from build123d import *

# Parameters (mm, degrees)
SKETCH1_R           = 11
BOSS_EXTRUDE1_DEPTH = 4
SKETCH5_R           = 5
SKETCH5_R_2         = 2
BOSS_EXTRUDE2_DEPTH = 15
SKETCH2_R           = 1.25
CUT_EXTRUDE1_DEPTH  = 10
SKETCH20_R          = 1.25
CUT_EXTRUDE2_DEPTH  = 4


with BuildPart() as part:
    # Sketch1 → Boss-Extrude1 (new body)
    with BuildSketch(Plane(origin=(0, 0, 0), x_dir=(1, 0, 0), z_dir=(0, 1, 0))):
        with Locations(Location((0, 0, 0), (0, 0, 270))):
            Circle(SKETCH1_R)
    extrude(amount=BOSS_EXTRUDE1_DEPTH)

    # Sketch5 → Boss-Extrude2 (add)
    with BuildSketch(Plane.XZ):
        with Locations(Location((0, 0, 0), (0, 0, 90))):
            Circle(SKETCH5_R)
        with Locations(Location((0, 0, 0), (0, 0, 270))):
            Circle(SKETCH5_R_2, mode=Mode.SUBTRACT)
    extrude(amount=BOSS_EXTRUDE2_DEPTH)

    # Sketch2 → Cut-Extrude1 (cut)
    with BuildSketch(Plane.XZ):
        with Locations(Location((0, -8, 0), (0, 0, 270))):
            Circle(SKETCH2_R)
        with Locations(Location((-8, 0, 0), (0, 0, 270))):
            Circle(SKETCH2_R)
        with Locations(Location((0, 8, 0), (0, 0, 270))):
            Circle(SKETCH2_R)
        with Locations(Location((8, 0, 0), (0, 0, 270))):
            Circle(SKETCH2_R)
    extrude(amount=-CUT_EXTRUDE1_DEPTH, mode=Mode.SUBTRACT)

    # Sketch20 → Cut-Extrude2 (cut)
    with BuildSketch(Plane(origin=(5, 0, 0), x_dir=(0, 0, -1), z_dir=(1, 0, 0))):
        with Locations((0, -4)):
            Circle(SKETCH20_R)
        with Locations((0, -11)):
            Circle(SKETCH20_R)
    extrude(amount=-CUT_EXTRUDE2_DEPTH, mode=Mode.SUBTRACT)


solid = part.part
The model under review builds one solid part; all positions refer to its coordinate system, in mm. A direction names the side the tool comes from. Give positions to 0.01 mm unless a question says otherwise; leave off trailing zeros. Loops run counter-clockwise (first coordinate to the right, second up) from the corner with the lowest first, then second, coordinate; pieces in that order, holes last. Notation, with made-up numbers: (55, 80) -> (72, 80) arc R20 ccw to (72, 107) -> close; hole circle Ø5 at (59.5, 32.5). An arc over 180 degrees is marked (long way). Answer as a JSON object with one key per item and string values. Group by question number.
Q1. Take a section at C-C (z = 8). Write out the cut boundary in (x, y).
Q2. Tool access review of faces 1 (the cylindrical face through (3.3, -10.95, 1.25)), 2 (the flat face through (0, 0, 0)), 3 (the flat face through (0, 4, 0)): name each direction out of +Z, -Z, +X, -X, +Y, -Y from which nothing blocks a thin tool from reaching the whole face with its end or side.
Q3. Take a section at A-A (x = 0). Write out the cut boundary in (y, z).
Q4. Draft analysis for pull direction Y (two halves, no side actions). For faces 4 (the cylindrical face through (0.05, 1.97, 9.25)), 5 (the cylindrical face through (3.3, -3.95, 1.25)), 6 (the flat face through (-0.1, -15, 2.2)), state which applies: pulls with the +Y half, pulls with the -Y half, needs draft (parallel to the pull), parting line crosses it, or undercut.
Q5. Take a section at B-B (x = 8). Write out the cut boundary in (y, z).
Q6. Insertion check: pin 1 (1.5 mm diameter, centred on y = -2.5, z = -1, fed in from -X); pin 2 (1.5 mm diameter, centred on x = 7, y = 1.5, fed in from +Z); pin 3 (3 mm diameter, centred on x = -8, z = 0, fed in from -Y); pin 4 (2 mm diameter, centred on x = 8, z = 0, fed in from +Y). Each pin has a flat end and moves straight along its axis. Give the tip position at first contact, or say it passes through.
Q7. Wall thickness on line 1 along X through (y, z) = (1.35, 0); line 2 along Y through (x, z) = (-6.5, 6.25); line 3 along X through (y, z) = (2.35, 8): over which ranges is each line inside the solid? List them lowest first.
Q8. Take a section at D-D (y = -7). Write out the cut boundary in (x, z).
Answer below:
{
 "1": {"outline": "(-7.55, 0) -> (-1.25, 0) -> (-1.25, 4) -> (-7.55, 4) -> close; (1.25, 0) -> (7.55, 0) -> (7.55, 4) -> (1.25, 4) -> close"},
 "2": {"face 1": "+X", "face 2": "-Y", "face 3": "+Z, -Z, +X, -X, +Y"},
 "3": {"outline": "(-15, -5) -> (0, -5) -> (0, -6.75) -> (4, -6.75) -> (4, 6.75) -> (0, 6.75) -> (0, 5) -> (-15, 5) -> (-15, 2) -> (0, 2) -> (0, -2) -> (-15, -2) -> close; (0, -11) -> (4, -11) -> (4, -9.25) -> (0, -9.25) -> close; (0, 9.25) -> (4, 9.25) -> (4, 11) -> (0, 11) -> close"},
 "4": {"face 4": "needs draft", "face 5": "undercut", "face 6": "pulls with the -Y half"},
 "5": {"outline": "(0, -7.55) -> (4, -7.55) -> (4, -1.25) -> (0, -1.25) -> close; (0, 1.25) -> (4, 1.25) -> (4, 7.55) -> (0, 7.55) -> close"},
 "6": {"pin 1": "stops at x = -4.99", "pin 2": "stops at z = 9.05", "pin 3": "stops at y = 0", "pin 4": "passes through"},
 "7": {"line 1": "x = -11 to -9.25, -6.75 to 6.75, 9.25 to 11", "line 2": "y = 0 to 4", "line 3": "x = -7.55 to -1.25, 1.25 to 7.55"},
 "8": {"outline": "circle Ø10 at (0, 0); hole circle Ø4 at (0, 0)"}
}
